from build123d import *

# Parameters (mm, degrees)
ESQUISSE1_W                     = 37.5
ESQUISSE1_H                     = 9.2
BOSS_EXTRU_1_DEPTH              = 2
CONG_1_R                        = 3
ESQUISSE2_R                     = 1
ENL_V_MAT_EXTRU_1_DEPTH         = 3
ESQUISSE3_W                     = 29.5
ESQUISSE3_H                     = 9.2
BOSS_EXTRU_2_DEPTH              = 4.551597138
CONG_2_R                        = 0.5
ESQUISSE4_W                     = 27.5
ESQUISSE4_H                     = 7.2
ENL_V_MAT_EXTRU_2_DEPTH         = 2
CONG_3_R                        = 2.5
ESQUISSE5_W                     = 13.7
ESQUISSE5_H                     = 5
BOSS_EXTRU_3_DEPTH              = 1
CONG_4_R                        = 1
ESQUISSE6_R                     = 0.75
BOSS_EXTRU_4_DEPTH              = 0.2
BOSS_EXTRU_5_START              = -5.751597
ESQUISSE7_R                     = 0.4
BOSS_EXTRU_5_DEPTH              = 1.758
R_P_TITION_LIN_AIRE1_COUNT      = 2
R_P_TITION_LIN_AIRE1_PITCH      = 2.54
R_P_TITION_LIN_AIRE1_COUNT_DIR2 = 5
R_P_TITION_LIN_AIRE1_PITCH_DIR2 = 2.54


with BuildPart() as part:
    # Esquisse1 → Boss.-Extru.1 (new body)
    with BuildSketch(Plane.XY):
        Rectangle(ESQUISSE1_W, ESQUISSE1_H)
    extrude(amount=BOSS_EXTRU_1_DEPTH)

    # Congé1
    cong_1_edges = [part.edges().sort_by_distance(p)[0] for p in [
        (-18.75, 4.6, 1),
        (18.75, 4.6, 1),
        (18.75, -4.6, 1),
        (-18.75, -4.6, 1),
    ]]
    fillet(cong_1_edges, radius=CONG_1_R)

    # Esquisse2 → Enlèv. mat.-Extru.1 (cut, through all)
    with BuildSketch(Plane.XY.offset(2)):
        with Locations((-16.75, 0)):
            Circle(ESQUISSE2_R)
    enl_v_mat_extru_1 = extrude(amount=-ENL_V_MAT_EXTRU_1_DEPTH, mode=Mode.SUBTRACT)

    # Symétrie1: Enlèv. mat.-Extru.1 across plane
    add(enl_v_mat_extru_1.mirror(Plane(origin=(0, 0, 0), x_dir=(0, 0, 1), z_dir=(1, 0, 0))), mode=Mode.SUBTRACT)

    # Esquisse3 → Boss.-Extru.2 (add)
    with BuildSketch(Plane.XY.offset(2)):
        Rectangle(ESQUISSE3_W, ESQUISSE3_H)
    extrude(amount=BOSS_EXTRU_2_DEPTH)

    # Congé2
    cong_2_edges = [part.edges().sort_by_distance(p)[0] for p in [
        (-14.75, 4.6, 4.275798569),
        (-14.75, -4.6, 4.275798569),
        (14.75, -4.6, 4.275798569),
        (14.75, 4.6, 4.275798569),
    ]]
    fillet(cong_2_edges, radius=CONG_2_R)

    # Esquisse4 → Enlèv. mat.-Extru.2 (cut)
    with BuildSketch(Plane.XY.offset(6.551597138)):
        Rectangle(ESQUISSE4_W, ESQUISSE4_H)
    extrude(amount=-ENL_V_MAT_EXTRU_2_DEPTH, mode=Mode.SUBTRACT)

    # Congé3
    cong_3_edges = [part.edges().sort_by_distance(p)[0] for p in [
        (13.75, 3.6, 5.551597138),
        (13.75, -3.6, 5.551597138),
    ]]
    fillet(cong_3_edges, radius=CONG_3_R)

    # Esquisse5 → Boss.-Extru.3 (add)
    with BuildSketch(Plane.XY.offset(4.551597138)):
        Rectangle(ESQUISSE5_W, ESQUISSE5_H)
    extrude(amount=BOSS_EXTRU_3_DEPTH)

    # Congé4
    cong_4_edges = [part.edges().sort_by_distance(p)[0] for p in [
        (-6.85, 2.5, 5.051597138),
        (-6.85, -2.5, 5.051597138),
        (6.85, -2.5, 5.051597138),
        (6.85, 2.5, 5.051597138),
    ]]
    fillet(cong_4_edges, radius=CONG_4_R)

    # Esquisse6 → Boss.-Extru.4 (add)
    with BuildSketch(Plane.XY.offset(5.551597138)):
        with Locations((-5.08, 1.27)):
            Circle(ESQUISSE6_R)
    boss_extru_4 = extrude(amount=BOSS_EXTRU_4_DEPTH)

    # Esquisse7 → Boss.-Extru.5 (add)
    with BuildSketch(Plane.XY.offset(5.751597138).offset(BOSS_EXTRU_5_START)):
        with Locations((-5.08, 1.27)):
            Circle(ESQUISSE7_R)
    boss_extru_5 = extrude(amount=-BOSS_EXTRU_5_DEPTH)

    # Répétition linéaire1: Boss.-Extru.4, Boss.-Extru.5 2 × 5
    with Locations(*[(j * R_P_TITION_LIN_AIRE1_PITCH_DIR2, -i * R_P_TITION_LIN_AIRE1_PITCH, 0) for i in range(R_P_TITION_LIN_AIRE1_COUNT) for j in range(R_P_TITION_LIN_AIRE1_COUNT_DIR2) if (i, j) != (0, 0)]):
        add(boss_extru_4)
        add(boss_extru_5)


solid = part.part
Read the model definition and answer for the solid it produces. Units are mm, in the model's axes. A direction names the side the tool comes from. Give positions to 0.01 mm unless a question says otherwise; leave off trailing zeros. Write each loop counter-clockwise with the first axis right and the second up, starting at its lowest first coordinate (ties: lowest second). Pieces come first, ordered by that corner, then holes. Notation, with made-up numbers: (23.25, 33.25) -> (53.25, 33.25) arc R13 ccw to (53.25, 51.25) -> close; hole circle Ø7 at (-40, 72.5). An arc over 180 degrees is marked (long way). Answer as a JSON object with one key per item and string values. Group by question number.
1) The mould has two halves that part along Y. Classify faces 4 (the cylindrical face through (-17.89, 3.7, 1.01)), 5 (the cylindrical face through (17.85, -3.74, 1.01)), 6 (the flat face through (0, 3, 4.552)): +Y half, -Y half, draft (parallel to the pull), parting line (faces both ways), or undercut.
2) Find section A-A (z = 5). Write down the section's boundary in (x, y).
3) Find section C-C (x = 16.75). Write down the section's boundary in (y, z).
4) Each of these flat-tipped pins is pushed along its axis until it touches: P1, Ø1.3, axis at x = -16.5, y = 0.5, coming from the +Z side; P2, Ø2.5, axis at y = -2, z = 5.5, coming from the -X side; P3, Ø1.2, axis at x = -5, y = 1, coming from the +Z side; P4, Ø1.8, axis at x = 16.75, y = 0, coming from the +Z side. Where does it stop, or does it pass through?
5) Consider L1, parallel to Y at x = 2.5, z = 6.25; L2, parallel to X at y = 0.5, z = 1; L3, parallel to Z at x = -15, y = -1.25. Determine where each line is inside the solid, lowest interval first. Write a range as from..to.
6) A tool of negligible diameter and unlimited length cuts with its end or side. For faces 1 (the flat face through (0, 1, 5.752)), 2 (the flat face through (14.75, 0, 4)), 3 (the cylindrical face through (4.68, -1.25, -0.87)), from which of +Z, -Z, +X, -X, +Y, -Y can it reach the whole face along a straight path? Write none if from no direction.
7) Find section D-D (x = 5.08). Write down the section's boundary in (y, z), and give its area (3 significant figures).
8) Find section B-B (z = 3). Write down the section's boundary in (x, y).
Values follow:
{
 "1": {"face 4": "+Y half", "face 5": "-Y half", "face 6": "undercut"},
 "2": {"outline": "(-14.75, -4.1) arc R0.5 ccw to (-14.25, -4.6) -> (14.25, -4.6) arc R0.5 ccw to (14.75, -4.1) -> (14.75, 4.1) arc R0.5 ccw to (14.25, 4.6) -> (-14.25, 4.6) arc R0.5 ccw to (-14.75, 4.1) -> close; (-6.85, -1.5) arc R1 ccw to (-5.85, -2.5) -> (5.85, -2.5) arc R1 ccw to (6.85, -1.5) -> (6.85, 1.5) arc R1 ccw to (5.85, 2.5) -> (-5.85, 2.5) arc R1 ccw to (-6.85, 1.5) -> close; hole (-13.75, -3.6) -> (11.25, -3.6) arc R2.5 ccw to (13.75, -1.1) -> (13.75, 1.1) arc R2.5 ccw to (11.25, 3.6) -> (-13.75, 3.6) -> close"},
 "3": {"outline": "(-4.43, 0) -> (-1, 0) -> (-1, 2) -> (-4.43, 2) -> close; (1, 0) -> (4.43, 0) -> (4.43, 2) -> (1, 2) -> close"},
 "4": {"P1": "stops at z = 2", "P2": "stops at x = -14.75", "P3": "stops at z = 5.75", "P4": "passes through"},
 "5": {"L1": "y = -4.6..-3.6, 3.6..4.6", "L2": "x = -18.75..-17.62, -15.88..15.88, 17.62..18.75", "L3": "z = 0..2"},
 "6": {"face 1": "+Z", "face 2": "+Z, +X, +Y, -Y", "face 3": "-Z"},
 "7": {"outline": "(-4.6, 0) -> (-1.67, 0) -> (-1.67, -1.76) -> (-0.87, -1.76) -> (-0.87, 0) -> (0.87, 0) -> (0.87, -1.76) -> (1.67, -1.76) -> (1.67, 0) -> (4.6, 0) -> (4.6, 6.55) -> (3.6, 6.55) -> (3.6, 4.55) -> (2.5, 4.55) -> (2.5, 5.55) -> (2.02, 5.55) -> (2.02, 5.75) -> (0.52, 5.75) -> (0.52, 5.55) -> (-0.52, 5.55) -> (-0.52, 5.75) -> (-2.02, 5.75) -> (-2.02, 5.55) -> (-2.5, 5.55) -> (-2.5, 4.55) -> (-3.6, 4.55) -> (-3.6, 6.55) -> (-4.6, 6.55) -> close", "area": "54.3 mm2"},
 "8": {"outline": "(-14.75, -4.1) arc R0.5 ccw to (-14.25, -4.6) -> (14.25, -4.6) arc R0.5 ccw to (14.75, -4.1) -> (14.75, 4.1) arc R0.5 ccw to (14.25, 4.6) -> (-14.25, 4.6) arc R0.5 ccw to (-14.75, 4.1) -> close"}
}
